Verification items for the finished model (mm, model axes). A direction names the side the tool comes from. Round coordinates to 2 decimals unless told otherwise and drop trailing zeros. Write each loop counter-clockwise with the first axis right and the second up, starting at its lowest first coordinate (ties: lowest second). Pieces come first, ordered by that corner, then holes. Notation, with made-up numbers: M 66.25,8.5 L 96.25,8.5 A29 ccw 96.25,45.5 Z; hole C 8.5,53 d11. An arc over 180 degrees is marked long. Use a Markdown table: item, result. Add a question column.
from build123d import *

# Parameters (mm, degrees)
F1_W          = 5.5
F1_H          = 5.5
F2_DEPTH      = 7
F2_DEPTH_BACK = 5.5
F3_W          = 5.5
F3_H          = 5.5
F4_DEPTH      = 5.5
F5_W          = 5.5
F5_H          = 5.5
F6_DEPTH      = 19.9
F8_DEPTH      = 2.75
F8_DEPTH_BACK = 2.75
F10_DEPTH     = 2.75


with BuildPart() as f2:
    # F1 (on Front) → F2 (new body, two sides)
    with BuildSketch(Plane.XZ) as f2_sk:
        Rectangle(F1_W, F1_H)
    extrude(amount=-F2_DEPTH)
    extrude(f2_sk.sketch, amount=F2_DEPTH_BACK)



with BuildPart() as f4:
    # F3 (on Front) → F4 (new body, through all)
    with BuildSketch(Plane.XZ):
        with Locations((0, 25.4)):
            Rectangle(F3_W, F3_H)
    extrude(amount=F4_DEPTH)


with BuildPart() as f2_1:
    add(f2.part)

    add(f4.part)  # F6 merges F4
    # F5 (on face) → F6 (join, through all)
    with BuildSketch(Plane.XY.offset(2.75)):
        with Locations((0, -2.75)):
            Rectangle(F5_W, F5_H)
    extrude(amount=F6_DEPTH)

    # F7 (on Right) → F8 (join, two sides)
    with BuildSketch(Plane.YZ) as f8_sk:
        Polygon((3.175, 28.15), (0, 28.15), (0, 22.65), (5.4531745931, 22.65), (12.5242424049, 29.7210678119), (8.6351551084, 33.6101551084), align=None)
    extrude(amount=F8_DEPTH)
    extrude(f8_sk.sketch, amount=-F8_DEPTH_BACK)

    # F9 (on Right) → F10 (join, symmetric)
    with BuildSketch(Plane.YZ):
        Polygon((0, -29.8453345895), (0, 0), (-5.5, 0), (-5.5, -15.6319836834), (-25.1807147937, 5.9900909129), (-28.2262068887, 5.4240246833), (-29.1399087291, 10.3398306206), (-38.8949113266, 21.0570934874), (-38.8949113266, 31.0857333243), (-44.3949113267, 31.0857333243), (-44.3949113267, 18.9288128167), align=None)
        Polygon((-28.2262068887, 5.4240246833), (-25.1807147937, 5.9900909129), (-29.1399087291, 10.3398306206), align=None)
        Polygon((-29.1399087291, 10.3398306206), (-25.1807147937, 5.9900909129), (-4.4631796137, 9.8408633531), (-5.3768814541, 14.7566692904), align=None)
    extrude(amount=F10_DEPTH, both=True)


solid = f2_1.part
1. Cross-section at C-C on y = -12. Enter the section's corners in (x, z).
2. Release check for a two-part mould opening along Z. For faces 1 (the flat face through (0, -1, 28.15)), 2 (the flat face through (0, 3, 22.65)), 3 (the flat face through (0, -5.5, -3)), 4 (the flat face through (0, 0, -16)) record: +Z half, -Z half, draft (parallel to the pull), parting line (faces both ways), or undercut.
3. Cross-section at B-B on z = 7. Enter the section's corners in (x, y), plus the area to 3 significant figures.
4. Scan lines: line 1 along Z through (x, y) = (-1.05, 3); line 2 along Z through (x, y) = (1, -8); line 3 along Y through (x, z) = (-2.5, 26). Record each from-to range of solid material in increasing order. Write a range as from..to.
5. Access from +Z, -Z, +X, -X, +Y, -Y to the whole of each face (thin tool, end or side, straight path). Record for faces 5 (the flat face through (0.038, 8.939, 26.136)), 6 (the flat face through (0.038, -15.478, 7.794)), 7 (the flat face through (0.038, -33.949, 15.623)).
6. Cross-section at A-A on x = -0.65. Enter the section's corners in (y, z) (3 decimals), plus the area to 3 significant figures.
7. Cross-section at D-D on y = -33.5. Enter the section's corners in (x, z).
8. Depth check by flat-ended pin: pin 1 Ø1.6 at (x, y) = (-1, 3.5) entering from +Z (3 decimals); pin 2 Ø1.6 at (x, z) = (1, 11) entering from +Y; pin 3 Ø1.6 at (x, y) = (0, 5) entering from -Z. Enter the tip coordinate at first touch or a pass-through.
Answer:
| question | item | result |
|---|---|---|
| 1 | outline | M -2.75,-16.66 L 2.75,-16.66 L 2.75,-8.49 L -2.75,-8.49 Z; M -2.75,8.44 L 2.75,8.44 L 2.75,13.53 L -2.75,13.53 Z |
| 2 | face 1 | +Z half |
| 2 | face 2 | undercut |
| 2 | face 3 | undercut |
| 2 | face 4 | draft |
| 3 | outline | M -2.75,-33.54 L 2.75,-33.54 L 2.75,-19.75 L -2.75,-19.75 Z; M -2.75,-5.5 L 2.75,-5.5 L 2.75,0 L -2.75,0 Z |
| 3 | area | 106 mm^2 |
| 4 | line 1 | z = -2.75..2.75, 22.65..28.15 |
| 4 | line 2 | z = -21.06..-12.89, 9.18..14.27 |
| 4 | line 3 | y = -44.39..-38.89, -5.5..8.8 |
| 5 | face 5 | +X, -X, +Y |
| 5 | face 6 | +X, -X |
| 5 | face 7 | +Z, +X, -X |
| 6 | outline | M -44.395,18.929 L 0,-29.845 L 0,-2.75 L 7,-2.75 L 7,2.75 L 0,2.75 L 0,22.65 L 5.453,22.65 L 12.524,29.721 L 8.635,33.61 L 3.175,28.15 L -5.5,28.15 L -5.5,14.734 L -29.14,10.34 L -38.895,21.057 L -38.895,31.086 L -44.395,31.086 Z; hole M -25.181,5.99 L -5.5,-15.632 L -5.5,9.648 Z |
| 6 | area | 880 mm^2 |
| 7 | outline | M -2.75,6.96 L 2.75,6.96 L 2.75,15.13 L -2.75,15.13 Z |
| 8 | pin 1 | stops at z = 29.275 |
| 8 | pin 2 | stops at y = 0 |
| 8 | pin 3 | stops at z = -2.75 |
